CAD build for the part. Positions are in the model's coordinates, mm. Face numbers are marked on the shaded views. A direction names the side the tool comes from. Round coordinates to 2 decimals unless told otherwise and drop trailing zeros. Order: outer loops, then holes, each group sorted by start corner. A loop starts at its lowest first (then second) coordinate and runs counter-clockwise, first axis right, second up.
```python
from build123d import *

# Parameters (mm, degrees)
BOSS_EXTRUDE1_DEPTH = 50
CUT_EXTRUDE1_DEPTH  = 48
SKETCH3_R           = 1.6
CUT_EXTRUDE2_DEPTH  = 840.282109633
FILLET3_R           = 1


with BuildPart() as part:
    # Sketch1 → Boss-Extrude1 (new body)
    with BuildSketch(Plane(origin=(0, 0, 0), x_dir=(1, 0, 0), z_dir=(0, 1, 0))):
        with BuildLine():
            Line((789.147942738, -65.404824394), (789.147942738, -25.404824394))
            Line((789.147942738, -25.404824394), (834.147942738, -25.404824394))
            Line((834.147942738, -25.404824394), (834.147942738, -37.404824394))
            Line((834.147942738, -37.404824394), (803.037942738, -37.404824394))
            Line((803.037942738, -37.404824394), (803.037942738, -58.807263418))
            Line((803.037942738, -58.807263418), (803.037942738, -79.294824394))
            ThreePointArc((803.037942738, -79.294824394), (793.216229548, -75.226537585), (789.147942738, -65.404824394))
        make_face()
    extrude(amount=BOSS_EXTRUDE1_DEPTH)

    # Sketch2 → Cut-Extrude1 (cut)
    with BuildSketch(Plane(origin=(0, 50, 0), x_dir=(1, 0, 0), z_dir=(0, 1, 0))):
        with BuildLine():
            Line((834.147942738, -27.404824394), (791.147942738, -27.404824394))
            Line((791.147942738, -27.404824394), (791.147942738, -65.404824394))
            ThreePointArc((791.147942738, -65.404824394), (794.630556885, -73.81166102), (803.037942738, -77.292949065))
            Line((803.037942738, -77.292949065), (834.147942738, -63.276412727))
            Line((834.147942738, -63.276412727), (834.147942738, -27.404824394))
        make_face()
    extrude(amount=-CUT_EXTRUDE1_DEPTH, mode=Mode.SUBTRACT)

    # Sketch3 → Cut-Extrude2 (cut, through all)
    with BuildSketch(Plane(origin=(0, 2, 0), x_dir=(1, 0, 0), z_dir=(0, 1, 0))):
        with Locations(Location((824.147942738, -32.904824394, 0), (0, 0, 270))):
            Circle(SKETCH3_R)
        with Locations(Location((796.647942738, -32.904824394, 0), (0, 0, 270))):
            Circle(SKETCH3_R)
        with Locations(Location((798.982858952, -70.344824394, 0), (0, 0, 270))):
            Circle(SKETCH3_R)
    extrude(amount=-CUT_EXTRUDE2_DEPTH, mode=Mode.SUBTRACT)

    # Fillet3
    fillet3_edges = [part.edges().sort_by_distance(p)[0] for p in [
        (794.630556885, 50, 73.81166102),
        (812.647942738, 50, 27.404824394),
        (791.147942738, 50, 46.404824394),
    ]]
    fillet(fillet3_edges, radius=FILLET3_R)


solid = part.part
```
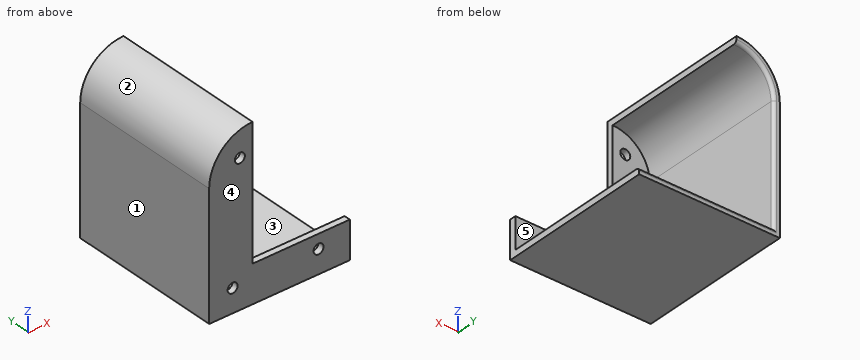
1. Cut at A-A, the plane y = 38. Write the cut outline in (x, z), and give its area (3 significant figures).
2. Pin check, flat tips, straight feed: P1, Ø1.5, axis at x = 797, y = 26, coming from the +Z side; P2, Ø1, axis at y = 20.5, z = 69.5, coming from the -X side; P3, Ø2, axis at x = 823, y = 1.5, coming from the +Z side. Stop position of each tip, or through.
3. Cut at C-C, the plane x = 807.5. Write the cut outline in (y, z), and give its area (3 significant figures).
4. Mould opens along Z. For the marked faces 1, 2 and 3 say: released by +Z, released by -Z, zero draft, split by the parting line, or undercut.
5. Drill centre lines: line 1 (Z direction, x = 823, y = 41); line 2 (X direction, y = 46, z = 28); line 3 (Z direction, x = 799, y = 28). Where is each one in solid material? Low to high.
6. Tool access for the marked faces 4 and 5: list every direction of +Z, -Z, +X, -X, +Y, -Y with a clear straight run to the whole face (end or side of a thin tool).
7. Cut at B-B, the plane z = 40. Write the cut outline in (x, y).
Outcome:
1. outline: (789.15, 25.4) - (834.15, 25.4) - (834.15, 27.4) - (791.15, 27.4) - (791.15, 65.4) arc R11.89 cw to (803.04, 77.29) - (803.04, 79.29) arc R13.89 ccw to (789.15, 65.4) - close
1. area: 207 mm2
2. P1: stops at z = 78.25
2. P2: stops at x = 789.62
2. P3: stops at z = 37.4
3. outline: (0, 25.4) - (50, 25.4) - (50, 26.4) arc R1 ccw to (49, 27.4) - (2, 27.4) - (2, 37.4) - (0, 37.4) - close
3. area: 120 mm2
4. face 1: zero draft
4. face 2: released by +Z
4. face 3: undercut
5. line 1: z = 25.4 to 27.4
5. line 2: x = 789.15 to 791.15
5. line 3: z = 25.4 to 27.4, 76.59 to 78.69
6. face 4: +Z, -Z, +X, -X, -Y
6. face 5: +X, +Y
7. outline: (789.15, 0) - (803.04, 0) - (803.04, 2) - (791.15, 2) - (791.15, 49) arc R1 ccw to (790.15, 50) - (789.15, 50) - close
